Model file for the job. Use its own axes, mm. A direction names the side the tool comes from. Round coordinates to 2 decimals unless told otherwise and drop trailing zeros. Order: outer loops, then holes, each group sorted by start corner. A loop starts at its lowest first (then second) coordinate and runs counter-clockwise, first axis right, second up. Notation, with made-up numbers: (19.5, -34) - (62.5, -34) arc R22 cw to (62.5, 3) - close; hole circle Ø11 at (27.25, 69.25). An arc over 180 degrees is marked (long way). Use one line per item in the form item = value.
from build123d import *

# Parameters (mm, degrees)
SKETCH2_R           = 7
SKETCH2_R_2         = 5
BOSS_EXTRUDE1_DEPTH = 1


with BuildPart() as part:
    # Sweep1: sweep along a path in Sketch1
    with BuildLine(Plane.ZY) as sweep1_path:
        Line((0, 0), (20, 0))
        Line((20, 0), (20, 30))
    # Sketch2 → Sweep1 (sweep)
    with BuildSketch(Plane.XY):
        Circle(SKETCH2_R)
        Circle(SKETCH2_R_2, mode=Mode.SUBTRACT)
    sweep(path=sweep1_path.line, transition=Transition.RIGHT)

    # Sketch3 → Boss-Extrude1 (add, symmetric)
    with BuildSketch(Plane(origin=(0, 0, 0), x_dir=(0, 0, -1), z_dir=(1, 0, 0))):
        Polygon((-13.456771137, 6.543228863), (-2.5, 6.543228863), (-13.456771137, 27.5), align=None)
    extrude(amount=BOSS_EXTRUDE1_DEPTH, both=True)


solid = part.part
(1) Probe probe 1 along Y at (x, z) = (0, 14.25); probe 2 along X at (y, z) = (2, 20); probe 3 along Y at (x, z) = (0, 6). List the from-to ranges inside material, lowest first. Write a range as [from, to].
Report:
probe_1 = [-7, -5], [5, 30]
probe_2 = [-7, -5], [5, 7]
probe_3 = [-7, -5], [5, 13.24]
(2) Slice it at D-D on y = 16. Give the cut face in (x, z).
Report:
outline = (-1, 7.44) - (1, 7.44) - (1, 13.07) arc R7 ccw (long way) to (-1, 13.07) - close; hole circle Ø10 at (0, 20)
(3) Slice it at C-C on z = 20. Give the cut face in (x, y).
Report:
outline = (-7, 0) arc R7 ccw to (7, 0) - (7, 30) - (5, 30) - (5, 0) arc R5 cw to (-5, 0) - (-5, 30) - (-7, 30) - close
(4) Slice it at A-A on x = -4.5. Give the cut face in (y, z), then the cut area to 3 significant figures.
Report:
outline = (-5.36, 0) - (-2.18, 0) - (-2.18, 22.18) - (30, 22.18) - (30, 25.36) - (-5.36, 25.36) - close; (2.18, 0) - (5.36, 0) - (5.36, 14.64) - (30, 14.64) - (30, 17.82) - (2.18, 17.82) - close
area = 318 mm2
(5) Pin check, flat tips, straight feed: pin 1 (5 mm diameter, centred on y = 19, z = 10, fed in from -X); pin 2 (1 mm diameter, centred on y = 11, z = 21.5, fed in from +X); pin 3 (2 mm diameter, centred on x = 5, z = 11.5, fed in from -Y); pin 4 (4 mm diameter, centred on x = 3, y = 3.5, fed in from -Z). Stop position of each tip, or through.
Report:
pin_1 = -1
pin_2 = 6.93
pin_3 = -5.74
pin_4 = 0
(6) Slice it at B-B on y = 0. Give the cut face in (x, z), then the cut area to 3 significant figures.
Report:
outline = (-7, 0) - (-5, 0) - (-5, 20) arc R5 cw to (5, 20) - (5, 0) - (7, 0) - (7, 20) arc R7 ccw to (-7, 20) - close
area = 118 mm2
(7) Pull direction Y, two halves, no side cores. Call faces 1 (the face through (-1.08, -4.88, 9.9)), 2 (the face through (5, 30, 18)), 3 (the face through (1, 13, 10)): released by +Y, released by -Y, zero draft, split by the parting line, or undercut.
Report:
face_1 = undercut
face_2 = released by +Y
face_3 = zero draft
(8) Tool access for faces 4 (the face through (-1, 13, 10)), 5 (the face through (-1.517, -6.834, 10.689)), 6 (the face through (-2, 5, 0)), 7 (the face through (-1.517, 15.87, 26.834)), 8 (the face through (0.014, 16.707, 7.814)): list every direction of +Z, -Z, +X, -X, +Y, -Y with a clear straight run to the whole face (end or side of a thin tool).
Report:
face_4 = -Z, -X, +Y
face_5 = -Z
face_6 = -Z, +X, -X, +Y, -Y
face_7 = +Y
face_8 = -Z, +X, -X, +Y
